For this review, use the dimensioned drawing (mm, ordinates from the lowest corner) and the shaded views. A direction names the side the tool comes from. Coordinates: 2 decimals unless noted, no trailing zeros. Write each loop counter-clockwise with the first axis right and the second up, starting at its lowest first coordinate (ties: lowest second). Pieces come first, ordered by that corner, then holes.
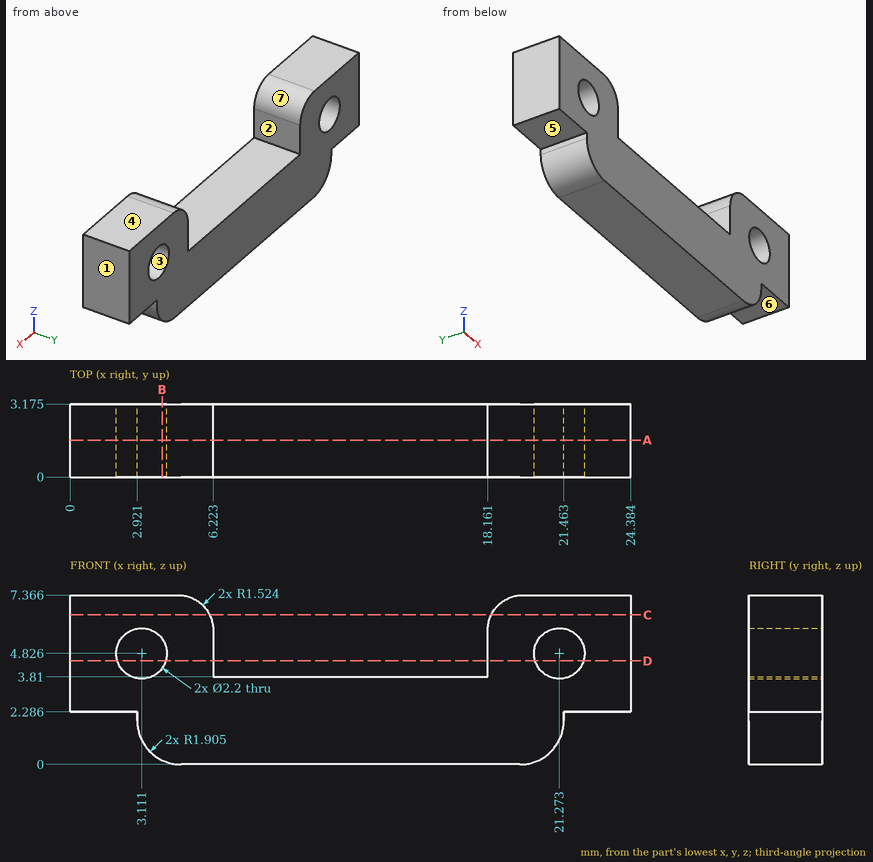
Item 1: Machinability: for the marked faces 5, 6 and 7, which of the approach directions +Z, -Z, +X, -X, +Y, -Y give a long, thin tool a straight path to every point of the face, cutting with its end or side? Answer none if there is none.
Solved:
face 5: -Z, -X, +Y, -Y
face 6: -Z, +X, +Y, -Y
face 7: +Z, +Y, -Y
Item 2: Take a section at A-A, the plane y = 1.6. Count the separate pieces of the cut face and the enclosed holes in it, plus the area to 3 significant figures.
Solved:
separate pieces: 1
enclosed holes: 2
area: 114 mm2
Item 3: Take a section at D-D, the plane z = 4.5. Write out the cut boundary in (x, y) (1 decimal).
Solved:
outline: (0, 0) - (2.1, 0) - (2.1, 3.2) - (0, 3.2) - close; (4.2, 0) - (6.2, 0) - (6.2, 3.2) - (4.2, 3.2) - close; (18.2, 0) - (20.2, 0) - (20.2, 3.2) - (18.2, 3.2) - close; (22.3, 0) - (24.4, 0) - (24.4, 3.2) - (22.3, 3.2) - close
Item 4: For pin 1 (1 mm diameter, centred on x = 14.5, y = 1.5, fed in from +Z); pin 2 (3.5 mm diameter, centred on x = 3.11, z = 4.83, fed in from -Y), all flat-tipped, find the tip position at first contact; note any pin that passes through.
Solved:
pin 1: stops at z = 3.81
pin 2: stops at y = 0
Item 5: To check wall thickness, follow line 1 along X through (y, z) = (2.75, 4.75) (1 decimal); line 2 along X through (y, z) = (1.5, 4) (1 decimal); line 3 along Z through (x, y) = (12.75, 2.15). State the ranges of each line that lie inside material, in increasing order.
Solved:
line 1: x = 0 to 2, 4.2 to 6.2, 18.2 to 20.2, 22.4 to 24.4
line 2: x = 0 to 2.4, 3.8 to 6.2, 18.2 to 20.5, 22 to 24.4
line 3: z = 0 to 3.81
Item 6: Mouldability with a two-part tool opening along X and no side actions: class the marked faces 1, 2, 3 and 4 as pulls with the +X half, pulls with the -X half, needs draft (parallel to the pull), parting line crosses it, or undercut.
Solved:
face 1: pulls with the +X half
face 2: undercut
face 3: undercut
face 4: needs draft
Item 7: Take a section at C-C, the plane z = 6.5. Write out the cut boundary in (x, y) (1 decimal).
Solved:
outline: (0, 0) - (6.1, 0) - (6.1, 3.2) - (0, 3.2) - close; (18.3, 0) - (24.4, 0) - (24.4, 3.2) - (18.3, 3.2) - close
Item 8: Take a section at B-B, the plane x = 4. Write out the cut boundary in (y, z) (1 decimal).
Solved:
outline: (0, 0.2) - (3.2, 0.2) - (3.2, 4.2) - (0, 4.2) - close; (0, 5.5) - (3.2, 5.5) - (3.2, 7.4) - (0, 7.4) - close
